from build123d import *

# Parameters (mm, degrees)
SKETCH1_R           = 2.5527
BOSS_EXTRUDE1_DEPTH = 50.00625


with BuildPart() as part:
    # Sketch1 → Boss-Extrude1 (new, symmetric)
    with BuildSketch(Plane(origin=(0, 0, 0), x_dir=(1, 0, 0), z_dir=(0, 1, 0))):
        with BuildLine():
            ThreePointArc((2.89465988, -6.35), (3.489325, -6.043688184), (4.051931374, -5.681848992))
            Line((4.051931374, -5.681848992), (6.946591254, -0.668151008))
            ThreePointArc((6.946591254, -0.668151008), (6.970630706, -0.334459838), (6.97865, 0))
            ThreePointArc((6.97865, 0), (6.970630706, 0.334459838), (6.946591254, 0.668151008))
            Line((6.946591254, 0.668151008), (4.051931374, 5.681848992))
            ThreePointArc((4.051931374, 5.681848992), (3.489325, 6.043688184), (2.89465988, 6.35))
            Line((2.89465988, 6.35), (-2.89465988, 6.35))
            ThreePointArc((-2.89465988, 6.35), (-3.489325, 6.043688184), (-4.051931374, 5.681848992))
            Line((-4.051931374, 5.681848992), (-6.946591254, 0.668151008))
            ThreePointArc((-6.946591254, 0.668151008), (-6.97865, 0), (-6.946591254, -0.668151008))
            Line((-6.946591254, -0.668151008), (-4.051931374, -5.681848992))
            ThreePointArc((-4.051931374, -5.681848992), (-3.489325, -6.043688184), (-2.89465988, -6.35))
            Line((-2.89465988, -6.35), (2.89465988, -6.35))
        make_face()
        with Locations(Location((0, 0, 0), (0, 0, 90))):
            Circle(SKETCH1_R, mode=Mode.SUBTRACT)
    extrude(amount=BOSS_EXTRUDE1_DEPTH, both=True)


solid = part.part
Source: CAD feature listing. Evaluate the final solid. Frame: model axes, mm. Give positions to 0.01 mm unless a question says otherwise; leave off trailing zeros. Write each loop counter-clockwise with the first axis right and the second up, starting at its lowest first coordinate (ties: lowest second). Pieces come first, ordered by that corner, then holes. Notation, with made-up numbers: (83.25, -2.75) - (131.25, -2.75) arc R19 ccw to (131.25, 16.25) - close; hole circle Ø6 at (-21, 78). An arc over 180 degrees is marked (long way). Write item = value, one per line. Start each with the question number.
Q1. Material intervals for probe 1 along X at (y, z) = (35, 1) (3 decimals); probe 2 along Z at (x, y) = (1, 42); probe 3 along Z at (x, y) = (1.25, 15), sorted ascending.
Q2. Cut plane C-C, the plane x = 5. Return loops of the section in (y, z).
Q3. Cut plane B-B, the plane x = 0. Return loops of the section in (y, z).
Q4. Pin query (flat end, axial travel): pin 1 Ø2 at (y, z) = (12, 3) entering from -X; pin 2 Ø8 at (x, y) = (5.5, 34) entering from -Z; pin 3 Ø2 at (y, z) = (21.5, -4.5) entering from +X; pin 4 Ø4 at (x, y) = (-5, -6.5) entering from +Z. Return the tip coordinate at first contact, or that it passes through.
Q5. Cut plane D-D, the plane z = 3.5. Return loops of the section in (x, y).
Q6. Cut plane A-A, the plane y = 32. Return loops of the section in (x, z).
Q7. Draft query along X for faces 1 (the cylindrical face through (-0.767, -0.7, -2.435)), 2 (the flat face through (0, 1, -6.35)), 3 (the flat face through (-5.52, 0.7, 3.14)), 4 (the flat face through (5.52, 0.7, -3.14)). Return one class per face: +X half, -X half, draft (parallel to the pull), parting line (faces both ways), or undercut.
Computed values:
q1.probe_1 = -6.755 to -2.349, 2.349 to 6.755
q1.probe_2 = -6.35 to -2.35, 2.35 to 6.35
q1.probe_3 = -6.35 to -2.23, 2.23 to 6.35
q2.outline = (-50.01, -4.04) - (50.01, -4.04) - (50.01, 4.04) - (-50.01, 4.04) - close
q3.outline = (-50.01, -6.35) - (50.01, -6.35) - (50.01, -2.55) - (-50.01, -2.55) - close; (-50.01, 2.55) - (50.01, 2.55) - (50.01, 6.35) - (-50.01, 6.35) - close
q4.pin_1 = -6.18
q4.pin_2 = -6.35
q4.pin_3 = 5.31
q4.pin_4 = 6.3
q5.outline = (-5.31, -50.01) - (5.31, -50.01) - (5.31, 50.01) - (-5.31, 50.01) - close
q6.outline = (-6.95, -0.67) - (-4.05, -5.68) arc R6.98 ccw to (-2.89, -6.35) - (2.89, -6.35) arc R6.98 ccw to (4.05, -5.68) - (6.95, -0.67) arc R6.98 ccw to (6.95, 0.67) - (4.05, 5.68) arc R6.98 ccw to (2.89, 6.35) - (-2.89, 6.35) arc R6.98 ccw to (-4.05, 5.68) - (-6.95, 0.67) arc R6.98 ccw to start; hole circle Ø5.11 at (0, 0)
q7.face_1 = undercut
q7.face_2 = draft
q7.face_3 = -X half
q7.face_4 = +X half
